from build123d import *

# Parameters (mm, degrees)
F1_DEPTH = 35
F2_DEPTH = 3
F3_W     = 9.7712434447
F3_H     = 18
F4_DEPTH = 12
F5_R     = 5


with BuildPart() as f1:
    # F0 (on Top) → F1 (new body)
    with BuildSketch(Plane.XY):
        with BuildLine():
            Line((-13.2287565553, 15), (-23, 15))
            Line((-23, 15), (-23, -23))
            Line((-23, -23), (23, -23))
            Line((23, -23), (23, 15))
            Line((23, 15), (13.2287565553, 15))
            ThreePointArc((13.2287565553, 15), (18.2287565553, 8.2287565553), (20, 0))
            ThreePointArc((20, 0), (-8.2287565553, -18.2287565553), (-13.2287565553, 15))
        make_face()
    extrude(amount=F1_DEPTH)

    # F0 (on Top) → F2 (join)
    with BuildSketch(Plane.XY):
        with BuildLine():
            Line((13.2287565553, 15), (-13.2287565553, 15))
            ThreePointArc((-13.2287565553, 15), (-8.2287565553, -18.2287565553), (20, 0))
            ThreePointArc((20, 0), (18.2287565553, 8.2287565553), (13.2287565553, 15))
        make_face()
    extrude(amount=F2_DEPTH)

    # F3 (on face) → F4 (cut)
    with BuildSketch(Plane(origin=(0, 15, 0), x_dir=(-1, 0, 0), z_dir=(0, 1, 0))):
        with Locations((-18.1143782777, 12)):
            Rectangle(F3_W, F3_H)
    extrude(amount=-F4_DEPTH, mode=Mode.SUBTRACT)

    # F5
    f5_edges = [f1.edges().sort_by_distance(p)[0] for p in [
        (21.38686, 3, 21),
        (21.38686, 3, 3),
    ]]
    fillet(f5_edges, radius=F5_R)


solid = f1.part
Design review of the part built by this model. Coordinates are the model's own, in mm. A direction names the side the tool comes from. Coordinates: 2 decimals unless noted, no trailing zeros. Loops run counter-clockwise (first coordinate to the right, second up) from the corner with the lowest first, then second, coordinate; pieces in that order, holes last. Notation, with made-up numbers: M -30.5,-21.5 L -6.5,-21.5 A20 ccw -6.5,-12.5 Z; hole C 79,-29 d10. An arc over 180 degrees is marked long. Use one line per item in the form item = value.
(1) Consider section A-A (z = 19.5). Write out the cut boundary in (x, y), and give its area (3 significant figures).
Return value:
outline = M -23,-23 L 23,-23 L 23,4.43 L 19.5,4.43 A20 cw long -13.23,15 L -23,15 Z
area = 520 mm2
(2) Consider section B-B (y = -17.5). Write out the cut boundary in (x, z).
Return value:
outline = M -23,0 L 23,0 L 23,35 L 9.68,35 L 9.68,3 L -9.68,3 L -9.68,35 L -23,35 Z
(3) For faces 1 (the face through (0, -4, 0)), 2 (the face through (21, 4, 19)), list the 3-axis set-ups (+Z, -Z, +X, -X, +Y, -Y) from which the entire face can be reached by the end or side of a thin tool; tool diameter is ignored.
Return value:
face_1 = -Z, +X, -X, +Y, -Y
face_2 = +X, +Y
(4) Draft analysis for pull direction Z (two halves, no side actions). For faces 3 (the face through (0, -21, 35)), 4 (the face through (21, 4, 5)), 5 (the face through (19, 12, 21)), 6 (the face through (18, 15, 28)), state which applies: pulls with the +Z half, pulls with the -Z half, needs draft (parallel to the pull), parting line crosses it, or undercut.
Return value:
face_3 = pulls with the +Z half
face_4 = undercut
face_5 = undercut
face_6 = needs draft
(5) Consider section C-C (x = -19). Write out the cut boundary in (y, z) (3 decimals), and give its area (3 significant figures).
Return value:
outline = M -23,0 L 15,0 L 15,35 L 6.245,35 L 6.245,3 L -6.245,3 L -6.245,35 L -23,35 Z
area = 930 mm2
(6) For line 1 along X through (y, z) = (0, 13); line 2 along Z through (x, y) = (-13, -1); line 3 along Y through (x, z) = (0, 20.5), list the stretches that pass through material, from the lowest coordinate up. Write a range as from..to.
Return value:
line_1 = -23..-20, 20..23
line_2 = 0..3
line_3 = -23..-20
(7) Consider section D-D (x = 0). Write out the cut boundary in (y, z), and give its area (3 significant figures).
Return value:
outline = M -23,0 L 15,0 L 15,3 L -20,3 L -20,35 L -23,35 Z
area = 210 mm2
(8) Clearance check with flat-ended pins moving along their axes: P1, Ø1, axis at x = 11.5, z = 8.5, coming from the +Y side; P2, Ø5, axis at x = 7.5, y = 10.5, coming from the +Z side; P3, Ø4, axis at x = 10.5, z = 14.5, coming from the +Y side. State where each tip first meets the part, or that it passes through.
Return value:
P1 = -16
P2 = 3
P3 = -15.61
